from build123d import *

# Parameters (mm, degrees)
F1_DEPTH     = 152.4
F2_DEPTH     = 12.7
F15_D        = 38.1
F15_ON_F13_D = 38.1
F15_ON_F12_D = 38.1
F15_ON_F11_D = 38.1
F15_ON_F10_D = 38.1
F15_ON_F9_D  = 38.1
F15_ON_F8_D  = 38.1
F15_ON_F7_D  = 38.1
F15_ON_F6_D  = 38.1
F15_ON_F5_D  = 38.1
F15_ON_F4_D  = 38.1
F15_ON_F3_D  = 38.1


with BuildPart() as f1:
    # F0 (on Top) → F1 (new body)
    with BuildSketch(Plane.XY):
        Polygon((98.6100561841, 368.0177398161), (0, 381), (-98.6100561841, 368.0177398161), (-190.5, 329.9556788419), (-269.4076836321, 269.4076836321), (-329.9556788419, 190.5), (-368.0177398161, 98.6100561841), (-381, 0), (-368.0177398161, -98.6100561841), (-329.9556788419, -190.5), (-269.4076836321, -269.4076836321), (-190.5, -329.9556788419), (-98.6100561841, -368.0177398161), (0, -381), (98.6100561841, -368.0177398161), (190.5, -329.9556788419), (269.4076836321, -269.4076836321), (329.9556788419, -190.5), (368.0177398161, -98.6100561841), (381, 0), (368.0177398161, 98.6100561841), (329.9556788419, 190.5), (269.4076836321, 269.4076836321), (190.5, 329.9556788419), align=None)
        Polygon((-95.2946909017, 355.6446281366), (0, 368.1904122006), (95.2946909017, 355.6446281366), (184.0952061003, 318.8622503956), (260.3499372349, 260.3499372349), (318.8622503956, 184.0952061003), (355.6446281366, 95.2946909017), (368.1904122006, 0), (355.6446281366, -95.2946909017), (318.8622503956, -184.0952061003), (260.3499372349, -260.3499372349), (184.0952061003, -318.8622503956), (95.2946909017, -355.6446281366), (0, -368.1904122006), (-95.2946909017, -355.6446281366), (-184.0952061003, -318.8622503956), (-260.3499372349, -260.3499372349), (-318.8622503956, -184.0952061003), (-355.6446281366, -95.2946909017), (-368.1904122006, 0), (-355.6446281366, 95.2946909017), (-318.8622503956, 184.0952061003), (-260.3499372349, 260.3499372349), (-184.0952061003, 318.8622503956), align=None, mode=Mode.SUBTRACT)
    extrude(amount=F1_DEPTH)

    # F0 (on Top) → F2 (join)
    with BuildSketch(Plane.XY):
        Polygon((95.2946909017, 355.6446281366), (0, 368.1904122006), (-95.2946909017, 355.6446281366), (-184.0952061003, 318.8622503956), (-260.3499372349, 260.3499372349), (-318.8622503956, 184.0952061003), (-355.6446281366, 95.2946909017), (-368.1904122006, 0), (-355.6446281366, -95.2946909017), (-318.8622503956, -184.0952061003), (-260.3499372349, -260.3499372349), (-184.0952061003, -318.8622503956), (-95.2946909017, -355.6446281366), (0, -368.1904122006), (95.2946909017, -355.6446281366), (184.0952061003, -318.8622503956), (260.3499372349, -260.3499372349), (318.8622503956, -184.0952061003), (355.6446281366, -95.2946909017), (368.1904122006, 0), (355.6446281366, 95.2946909017), (318.8622503956, 184.0952061003), (260.3499372349, 260.3499372349), (184.0952061003, 318.8622503956), align=None)
    extrude(amount=F2_DEPTH)

    # F15 (through all)
    with Locations(Plane(origin=(49.305028092, 374.5088699081, 0), x_dir=(-0.9914448614, 0.1305261922, 0), z_dir=(0.1305261922, 0.9914448614, 0))):
        with Locations((0, 102.6695207642)):
            Hole(F15_D / 2)

    # F15 on F13 (through all)
    with Locations(Plane(origin=(144.555028092, 348.986709329, 0), x_dir=(-0.9238795325, 0.3826834324, 0), z_dir=(0.3826834324, 0.9238795325, 0))):
        with Locations((0, 102.6695207642)):
            Hole(F15_ON_F13_D / 2)

    # F15 on F12 (through all)
    with Locations(Plane(origin=(229.953841816, 299.681681237, 0), x_dir=(-0.7933533403, 0.608761429, 0), z_dir=(0.608761429, 0.7933533403, 0))):
        with Locations((0, 102.6695207642)):
            Hole(F15_ON_F12_D / 2)

    # F15 on F11 (through all)
    with Locations(Plane(origin=(299.681681237, 229.953841816, 0), x_dir=(-0.608761429, 0.7933533403, 0), z_dir=(0.7933533403, 0.608761429, 0))):
        with Locations((0, 102.6695207642)):
            Hole(F15_ON_F11_D / 2)

    # F15 on F10 (through all)
    with Locations(Plane(origin=(348.986709329, 144.555028092, 0), x_dir=(-0.3826834324, 0.9238795325, 0), z_dir=(0.9238795325, 0.3826834324, 0))):
        with Locations((0, 102.6695207642)):
            Hole(F15_ON_F10_D / 2)

    # F15 on F9 (through all)
    with Locations(Plane(origin=(374.5088699081, 49.305028092, 0), x_dir=(-0.1305261922, 0.9914448614, 0), z_dir=(0.9914448614, 0.1305261922, 0))):
        with Locations((0, 102.6695207642)):
            Hole(F15_ON_F9_D / 2)

    # F15 on F8 (through all)
    with Locations(Plane(origin=(374.5088699081, -49.305028092, 0), x_dir=(0.1305261922, 0.9914448614, 0), z_dir=(0.9914448614, -0.1305261922, 0))):
        with Locations((0, 102.6695207642)):
            Hole(F15_ON_F8_D / 2)

    # F15 on F7 (through all)
    with Locations(Plane(origin=(348.986709329, -144.555028092, 0), x_dir=(0.3826834324, 0.9238795325, 0), z_dir=(0.9238795325, -0.3826834324, 0))):
        with Locations((0, 102.6695207642)):
            Hole(F15_ON_F7_D / 2)

    # F15 on F6 (through all)
    with Locations(Plane(origin=(299.681681237, -229.953841816, 0), x_dir=(0.608761429, 0.7933533403, 0), z_dir=(0.7933533403, -0.608761429, 0))):
        with Locations((0, 102.6695207642)):
            Hole(F15_ON_F6_D / 2)

    # F15 on F5 (through all)
    with Locations(Plane(origin=(229.953841816, -299.681681237, 0), x_dir=(0.7933533403, 0.608761429, 0), z_dir=(0.608761429, -0.7933533403, 0))):
        with Locations((0, 102.6695207642)):
            Hole(F15_ON_F5_D / 2)

    # F15 on F4 (through all)
    with Locations(Plane(origin=(144.555028092, -348.986709329, 0), x_dir=(0.9238795325, 0.3826834324, 0), z_dir=(0.3826834324, -0.9238795325, 0))):
        with Locations((0, 102.6695207642)):
            Hole(F15_ON_F4_D / 2)

    # F15 on F3 (through all)
    with Locations(Plane(origin=(49.305028092, -374.5088699081, 0), x_dir=(0.9914448614, 0.1305261922, 0), z_dir=(0.1305261922, -0.9914448614, 0))):
        with Locations((0, 102.6695207642)):
            Hole(F15_ON_F3_D / 2)


solid = f1.part
Read the model definition and answer for the solid it produces. Units are mm, in the model's axes. A direction names the side the tool comes from. Give positions to 0.01 mm unless a question says otherwise; leave off trailing zeros. Answer as CSV lines item,"result".
Item 1: Consider line 1 (Z direction, x = 142.5, y = -33.5); line 2 (X direction, y = -97, z = 62); line 3 (Y direction, x = -81, z = 88). Determine where each line is inside the solid, lowest interval first. Write a range as [from, to].
Returned:
line 1,"z = [0, 12.7]"
line 2,"x = [-368.23, -354.94], [354.94, 368.23]"
line 3,"y = [-370.34, -357.53], [357.53, 370.34]"
Item 2: For faces 1 (the face through (300.106, 229.401, 75.133)), 2 (the face through (139.1, 337.5, 81.6)), determine the directions among +Z, -Z, +X, -X, +Y, -Y from which every point of the face is accessible in a straight line to the end or side of a thin tool.
Returned:
face 1,"+Z, -Z, +X, +Y"
face 2,"+Z"
Item 3: Determine the mould class of faces 3 (the face through (-143.912, 349.253, 75.133)), 4 (the face through (-289.197, -222.756, 81.572)), 5 (the face through (-49.995, -374.418, 75.133)) for opening direction Y: +Y half, -Y half, draft (parallel to the pull), parting line (faces both ways), or undercut.
Returned:
face 3,"+Y half"
face 4,"undercut"
face 5,"-Y half"
Item 4: Each of these flat-tipped pins is pushed along its axis until it touches: pin 1 (10 mm diameter, centred on x = -144.5, z = 123.5, fed in from -Y); pin 2 (10 mm diameter, centred on y = -38, z = 94, fed in from -X); pin 3 (1.5 mm diameter, centred on y = 147, z = 32, fed in from +X). Where does it stop, or does it pass through?
Returned:
pin 1,"stops at y = -351.08"
pin 2,"stops at x = -376.64"
pin 3,"stops at x = 348.28"
Item 5: Find section A-A on y = -227.5. State how many separate pieces and enclosed holes the cut face has, plus the area to 3 significant figures.
Returned:
separate pieces,"3"
enclosed holes,"0"
area,"10,900 mm²"
